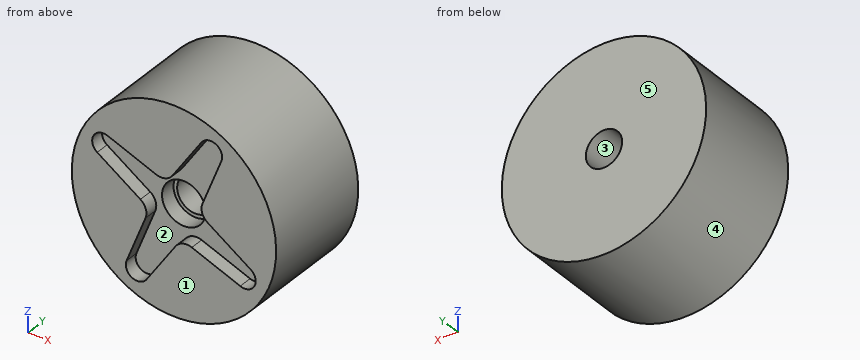
```python
from build123d import *

# Parameters (mm, degrees)
ESQUISSE1_R              = 22.5
ESQUISSE1_R_2            = 4
BOSS_EXTRU_1_DEPTH       = 25
EMPREINTE2_OUTLINE_R     = 4
EMPREINTE2_DEPTH         = 3
EMPREINTE2_START         = 3
EMPREINTE2_2_OUTLINE_R   = 4.8
EMPREINTE2_2_OUTLINE_R_2 = 4
EMPREINTE2_2_DEPTH       = 3.5


# Read off the part's stored shape, not the designer's step: Empreinte2
with BuildPart() as part:
    # Esquisse1 → Boss.-Extru.1 (new body)
    with BuildSketch(Plane(origin=(0, 0, 0), x_dir=(1, 0, 0), z_dir=(0, 1, 0))):
        with Locations(Location((0, 0, 0), (0, 0, 270))):
            Circle(ESQUISSE1_R)
        with Locations(Location((0, 0, 0), (0, 0, 270))):
            Circle(ESQUISSE1_R_2, mode=Mode.SUBTRACT)
    extrude(amount=BOSS_EXTRU_1_DEPTH)

    # Empreinte2 outline → Empreinte2 (cut)
    with BuildSketch(Plane(origin=(0, 0, 0), x_dir=(1, 0, 0), z_dir=(0, 1, 0))):
        with BuildLine():
            ThreePointArc((16.901774097, 6.031934529), (17.724046015, 9.265969613), (14.599132464, 10.436452132))
            Line((14.599132464, 10.436452132), (3.932151869, 6.270816496))
            ThreePointArc((3.932151869, 6.270816496), (1.943748033, 6.202567499), (0.349915852, 7.393410359))
            Line((0.349915852, 7.393410359), (-6.031934529, 16.901774097))
            ThreePointArc((-6.031934529, 16.901774097), (-9.265969613, 17.724046015), (-10.436452132, 14.599132464))
            Line((-10.436452132, 14.599132464), (-6.270816496, 3.932151869))
            ThreePointArc((-6.270816496, 3.932151869), (-6.202567499, 1.943748033), (-7.393410359, 0.349915852))
            Line((-7.393410359, 0.349915852), (-16.901774097, -6.031934529))
            ThreePointArc((-16.901774097, -6.031934529), (-17.724046015, -9.265969613), (-14.599132464, -10.436452132))
            Line((-14.599132464, -10.436452132), (-3.932151869, -6.270816496))
            ThreePointArc((-3.932151869, -6.270816496), (-1.943748033, -6.202567499), (-0.349915852, -7.393410359))
            Line((-0.349915852, -7.393410359), (6.031934529, -16.901774097))
            ThreePointArc((6.031934529, -16.901774097), (9.265969613, -17.724046015), (10.436452132, -14.599132464))
            Line((10.436452132, -14.599132464), (6.270816496, -3.932151869))
            ThreePointArc((6.270816496, -3.932151869), (6.202567499, -1.943748033), (7.393410359, -0.349915852))
            Line((7.393410359, -0.349915852), (16.901774097, 6.031934529))
        make_face()
        Circle(EMPREINTE2_OUTLINE_R, mode=Mode.SUBTRACT)
    extrude(amount=EMPREINTE2_DEPTH, mode=Mode.SUBTRACT)

    # Empreinte2 2 outline → Empreinte2 2 (cut)
    with BuildSketch(Plane(origin=(0, 0, 0), x_dir=(1, 0, 0), z_dir=(0, 1, 0)).offset(EMPREINTE2_START)):
        Circle(EMPREINTE2_2_OUTLINE_R)
        Circle(EMPREINTE2_2_OUTLINE_R_2, mode=Mode.SUBTRACT)
    extrude(amount=EMPREINTE2_2_DEPTH, mode=Mode.SUBTRACT)


solid = part.part
```
Input: part model. Units: mm. Frame: model coordinates. Face numbers are marked on the shaded views. A direction names the side the tool comes from. Give positions to 0.01 mm unless a question says otherwise; leave off trailing zeros. Order: outer loops, then holes, each group sorted by start corner. A loop starts at its lowest first (then second) coordinate and runs counter-clockwise, first axis right, second up. Notation, with made-up numbers: (76.25, 63.5) - (111.25, 63.5) arc R20 cw to (111.25, 89.5) - close; hole circle Ø10 at (58, 81.5). An arc over 180 degrees is marked (long way). One line per item, written item: value.
1. Cut plane D-D, the plane x = -8.5. Output: boundary loops of the cut face in (y, z), and give its area (3 significant figures).
Determined:
outline: (0, -20.83) - (25, -20.83) - (25, 20.83) - (0, 20.83) - (0, 8.05) - (3, 8.05) - (3, 0.39) - (0, 0.39) - (0, -9.64) - (3, -9.64) - (3, -17.98) - (0, -17.98) - close
area: 994 mm2
2. Cut plane C-C, the plane z = -1.5. Output: boundary loops of the cut face in (x, y), and give its area (3 significant figures).
Determined:
outline: (-22.45, 0) - (-6.38, 0) - (-6.38, 3) - (-4.56, 3) - (-4.56, 6.5) - (-3.71, 6.5) - (-3.71, 25) - (-22.45, 25) - close; (3.71, 6.5) - (4.56, 6.5) - (4.56, 3) - (10.15, 3) - (10.15, 0) - (22.45, 0) - (22.45, 25) - (3.71, 25) - close
area: 904 mm2
3. Draft query along X for the marked faces 3, 4 and 5. Return one class per face: released by +X, released by -X, zero draft, split by the parting line, or undercut.
Determined:
face 3: undercut
face 4: split by the parting line
face 5: zero draft
4. Cut plane A-A, the plane x = -2.5. Output: boundary loops of the cut face in (y, z), and give its area (3 significant figures).
Determined:
outline: (0, -22.36) - (25, -22.36) - (25, -3.12) - (6.5, -3.12) - (6.5, -4.1) - (3, -4.1) - (3, -11.64) - (0, -11.64) - close; (0, 6.08) - (3, 6.08) - (3, 4.1) - (6.5, 4.1) - (6.5, 3.12) - (25, 3.12) - (25, 22.36) - (0, 22.36) - close
area: 921 mm2
5. Cut plane B-B, the plane y = 2. Output: boundary loops of the cut face in (x, z).
Determined:
outline: circle Ø45 at (0, 0); hole (-16.9, 6.03) - (-7.39, -0.35) arc R3 cw to (-6.27, -3.93) - (-10.44, -14.6) arc R2.5 ccw to (-6.03, -16.9) - (0.35, -7.39) arc R3 cw to (3.93, -6.27) - (14.6, -10.44) arc R2.5 ccw to (16.9, -6.03) - (7.39, 0.35) arc R3 cw to (6.27, 3.93) - (10.44, 14.6) arc R2.5 ccw to (6.03, 16.9) - (-0.35, 7.39) arc R3 cw to (-3.93, 6.27) - (-14.6, 10.44) arc R2.5 ccw to start
6. Line query: probe 1 along X at (y, z) = (11.5, 0); probe 2 along X at (y, z) = (4.3, 0); probe 3 along Z at (x, y) = (-1.5, 2). Output: solid intervals per line, ascending.
Determined:
probe 1: -22.5 to -4, 4 to 22.5
probe 2: -22.5 to -4.8, 4.8 to 22.5
probe 3: -22.45 to -10.15, 6.38 to 22.45
7. Reachability of the marked faces 1 and 2 from +Z, -Z, +X, -X, +Y, -Y: full face, straight path, thin tool, end or side. Return the list, or none.
Determined:
face 1: +Z, -Z, +X, -X, -Y
face 2: -Y
8. Pin query (flat end, axial travel): pin 1 Ø6 at (x, y) = (-14.5, 6) entering from -Z; pin 2 Ø6 at (x, z) = (0, 0) entering from +Y; pin 3 Ø3 at (x, y) = (16, 13) entering from +Z; pin 4 Ø10.5 at (x, z) = (0, 0) entering from -Y. Return the tip coordinate at first contact, or that it passes through.
Determined:
pin 1: z = -19.34
pin 2: through
pin 3: z = 17.2
pin 4: y = 3
